from build123d import *

# Parameters (mm, degrees)
EXTRUDE_THIN1_DEPTH = 15
SKETCH2_OUTSIDE_W   = 38.632
SKETCH2_OUTSIDE_H   = 40.272
SKETCH2_OUTSIDE_R   = 13.3
SKETCH2_OUTSIDE_R_2 = 9.9
EXTRUDE1_DEPTH      = 30


with BuildPart() as part:
    # Sketch1 → Extrude-Thin1 (new, symmetric)
    with BuildSketch(Plane.XY):
        with BuildLine():
            ThreePointArc((14, 0), (10.511476834, -1.679487802), (6.646471406, -1.907974583))
            Line((6.646471406, -1.907974583), (-6.646471406, -0.092025417))
            ThreePointArc((-6.646471406, -0.092025417), (-10.511476834, -0.320512198), (-14, -2))
            Line((-14, -2), (-13.64, -2.48))
            ThreePointArc((-13.64, -2.48), (-10.360788224, -0.901281466), (-6.727683122, -0.686503892))
            Line((-6.727683122, -0.686503892), (6.565259691, -2.502453058))
            ThreePointArc((6.565259691, -2.502453058), (10.662165444, -2.26025707), (14.36, -0.48))
            Line((14.36, -0.48), (14, 0))
        make_face()
    extrude(amount=EXTRUDE_THIN1_DEPTH, both=True)

    # Sketch2 outside → Extrude1 (cut)
    # profile 1 of 2: a face of its own
    with BuildSketch(Plane(origin=(0, 0, 0), x_dir=(1, 0, 0), z_dir=(0, 1, 0))):
        with Locations((0.18, 0)):
            Rectangle(SKETCH2_OUTSIDE_W, SKETCH2_OUTSIDE_H)
        with Locations(Location((0, 0, 0), (0, 0, 299.579355848))):
            Circle(SKETCH2_OUTSIDE_R, mode=Mode.SUBTRACT)
    # profile 2 of 2: a face of its own
    with BuildSketch(Plane(origin=(0, 0, 0), x_dir=(1, 0, 0), z_dir=(0, 1, 0))):
        with Locations(Location((0, 0, 0), (0, 0, 311.541132012))):
            Circle(SKETCH2_OUTSIDE_R_2)
    extrude(amount=-EXTRUDE1_DEPTH, mode=Mode.SUBTRACT)


solid = part.part
Could you check a few things on this model? Use its own coordinates, in mm. Give positions to 0.01 mm unless a question says otherwise; leave off trailing zeros. Order: outer loops, then holes, each group sorted by start corner. A loop starts at its lowest first (then second) coordinate and runs counter-clockwise, first axis right, second up. Notation, with made-up numbers: (34, -21.5) - (72, -21.5) arc R23 ccw to (72, 4.5) - close; hole circle Ø1 at (6, 28). An arc over 180 degrees is marked (long way). Return JSON: item names as keys, results as strings. Group by question number.
Q1. Please list where these lines run through material, in increasing order: line 1 along Z through (x, y) = (0, -1.5); line 2 along Z through (x, y) = (2.25, -1.4); line 3 along Y through (x, z) = (-12, -0.25). Write a range as [from, to].
Q2. Suppose I cut it at B-B, the plane x = 0.5. Please give me the cut outline in (y, z), and give its area (3 significant figures).
Q3. Suppose I cut it at D-D, the plane x = -10.5. Please give me the cut outline in (y, z), and give its area (3 significant figures).
Q4. Suppose I cut it at A-A, the plane z = -3.5. Please give me the cut outline in (x, y) (3 decimals).
Q5. Suppose I cut it at C-C, the plane z = -10.25. Please give me the cut outline in (x, y), and give its area (3 significant figures).
Q6. Thinking about a two-plate mould opening in X: for faces 1 (the face through (-1.065, -1.297, 13.257)), 2 (the face through (10.146, -1.767, 0.161)), which applies, pulls with the +X half, pulls with the -X half, needs draft (parallel to the pull), parting line crosses it, or undercut?
Q7. Will these pins go through, and if not, where does the flat tip stop? pin 1 Ø1 at (x, y) = (5.5, -2) entering from +Z; pin 2 Ø1.5 at (x, z) = (-8.5, 4.5) entering from +Y; pin 3 Ø3 at (x, z) = (-10, 2.5) entering from +Y.
Resolved:
{
 "1": {"line 1": "z = [-13.3, -9.9], [9.9, 13.3]", "line 2": "z = [-13.11, -9.64], [9.64, 13.11]", "line 3": "y = [-1.49, -0.83]"},
 "2": {"outline": "(-1.67, -13.29) - (-1.07, -13.29) - (-1.07, -9.89) - (-1.67, -9.89) - close; (-1.67, 9.89) - (-1.07, 9.89) - (-1.07, 13.29) - (-1.67, 13.29) - close", "area": "4.12 mm2"},
 "3": {"outline": "(-0.94, -8.16) - (-0.32, -8.16) - (-0.32, 8.16) - (-0.94, 8.16) - close", "area": "10.1 mm2"},
 "4": {"outline": "(-12.831, -1.937) arc R9.4 cw to (-9.261, -0.685) - (-9.261, -0.08) arc R10 ccw to (-12.831, -1.244) - close; (9.261, -2.525) arc R10.6 ccw to (12.831, -1.435) - (12.831, -0.756) arc R10 cw to (9.261, -1.92) - close"},
 "5": {"outline": "(-8.48, -0.61) arc R9.4 cw to (-6.73, -0.69) - (6.57, -2.5) arc R10.6 ccw to (8.48, -2.59) - (8.48, -1.99) arc R10 cw to (6.65, -1.91) - (-6.65, -0.09) arc R10 ccw to (-8.48, -0.01) - close", "area": "10.2 mm2"},
 "6": {"face 1": "parting line crosses it", "face 2": "undercut"},
 "7": {"pin 1": "stops at z = 12.32", "pin 2": "stops at y = -0.01", "pin 3": "stops at y = -0.07"}
}
